```python
from build123d import *

# Parameters (mm, degrees)
F0_W      = 14
F0_H      = 58
F1_DEPTH  = 5
F3_DEPTH  = 25
F5_W      = 23
F5_H      = 3.5
F6_DEPTH  = 19.5
F7_W      = 14
F7_H      = 5
F8_DEPTH  = 8
F10_DEPTH = 12


with BuildPart() as f1:
    # F0 (on Top) → F1 (new body)
    with BuildSketch(Plane.XY):
        with Locations((7, 29)):
            Rectangle(F0_W, F0_H)
    extrude(amount=F1_DEPTH)

    # F2 (on face) → F3 (cut)
    with BuildSketch(Plane.XY.offset(5)):
        with BuildLine():
            ThreePointArc((8.5, 26.9), (8.0606601718, 27.9606601718), (7, 28.4))
            Line((7, 28.4), (7, 26.9))
            Line((7, 26.9), (8.5, 26.9))
        make_face()
        with BuildLine():
            Line((7, 26.9), (7, 28.4))
            ThreePointArc((7, 28.4), (5.9393398282, 27.9606601718), (5.5, 26.9))
            Line((5.5, 26.9), (7, 26.9))
        make_face()
        with BuildLine():
            Line((7, 25.4), (7, 26.9))
            Line((7, 26.9), (5.5, 26.9))
            ThreePointArc((5.5, 26.9), (5.9393398282, 25.8393398282), (7, 25.4))
        make_face()
        with BuildLine():
            Line((8.5, 26.9), (7, 26.9))
            Line((7, 26.9), (7, 25.4))
            ThreePointArc((7, 25.4), (8.0606601718, 25.8393398282), (8.5, 26.9))
        make_face()
        with BuildLine():
            ThreePointArc((8.5, 6.6), (8.0606601718, 7.6606601718), (7, 8.1))
            Line((7, 8.1), (7, 6.6))
            Line((7, 6.6), (8.5, 6.6))
        make_face()
        with BuildLine():
            Line((7, 6.6), (7, 8.1))
            ThreePointArc((7, 8.1), (5.9393398282, 5.5393398282), (8.5, 6.6))
            Line((8.5, 6.6), (7, 6.6))
        make_face()
    extrude(amount=-F3_DEPTH, mode=Mode.SUBTRACT)

    # F5 (on offset) → F6 (join)
    with BuildSketch(Plane(origin=(0, 55.5, 0), x_dir=(-1, 0, 0), z_dir=(0, 1, 0))):
        with Locations((-7, 10.25)):
            Rectangle(F5_W, F5_H)
        Polygon((-18.5, 0), (0, 0), (4.5, 0), (4.5, 8.5), (-18.5, 8.5), align=None)
    extrude(amount=-F6_DEPTH)

    # F7 (on face) → F8 (cut)
    with BuildSketch(Plane(origin=(0, 58, 0), x_dir=(-1, 0, 0), z_dir=(0, 1, 0))):
        with Locations((-7, 2.5)):
            Rectangle(F7_W, F7_H)
        Polygon((-18.5, 0), (-14, 0), (-14, 5), (0, 5), (0, 8.5), (-18.5, 8.5), align=None)
        Polygon((0, 5), (0, 0), (4.5, 0), (4.5, 8.5), (0, 8.5), align=None)
        Polygon((-18.5, 8.5), (0, 8.5), (4.5, 8.5), (4.5, 12), (-18.5, 12), align=None)
    extrude(amount=-F8_DEPTH, mode=Mode.SUBTRACT)

    # F9 (on face) → F10 (cut)
    with BuildSketch(Plane(origin=(0, 50, 0), x_dir=(-1, 0, 0), z_dir=(0, 1, 0))):
        with BuildLine():
            ThreePointArc((-10, 6), (-10.3661165235, 6.8838834765), (-11.25, 7.25))
            Line((-11.25, 7.25), (-11.25, 6))
            Line((-11.25, 6), (-12.5, 6))
            ThreePointArc((-12.5, 6), (-11.25, 4.75), (-10, 6))
        make_face()
        with BuildLine():
            Line((-11.25, 6), (-11.25, 7.25))
            ThreePointArc((-11.25, 7.25), (-12.1338834765, 6.8838834765), (-12.5, 6))
            Line((-12.5, 6), (-11.25, 6))
        make_face()
        with BuildLine():
            ThreePointArc((-1.5, 6), (-1.8661165235, 6.8838834765), (-2.75, 7.25))
            Line((-2.75, 7.25), (-2.75, 6))
            Line((-2.75, 6), (-1.5, 6))
        make_face()
        with BuildLine():
            Line((-2.75, 6), (-2.75, 7.25))
            ThreePointArc((-2.75, 7.25), (-3.6338834765, 5.1161165235), (-1.5, 6))
            Line((-1.5, 6), (-2.75, 6))
        make_face()
    extrude(amount=-F10_DEPTH, mode=Mode.SUBTRACT)


solid = f1.part
```
Geometry: final body of the model. Coordinates: model frame, mm. A direction names the side the tool comes from. Round coordinates to 2 decimals unless told otherwise and drop trailing zeros. Order: outer loops, then holes, each group sorted by start corner. A loop starts at its lowest first (then second) coordinate and runs counter-clockwise, first axis right, second up. Notation, with made-up numbers: (89, 70) -> (140, 70) arc R16 cw to (140, 95) -> close; hole circle Ø7 at (0.5, 21). An arc over 180 degrees is marked (long way). Use one line per item in the form item = value.
(1) Ray query, probe 1 along X at (y, z) = (46.5, 6); probe 2 along Y at (x, z) = (7, 2.25); probe 3 along Z at (x, y) = (2.75, 41.5). Return the intervals inside material, ascending. Write a range as [from, to].
Results list:
probe_1 = [-4.5, 1.5], [4, 10], [12.5, 18.5]
probe_2 = [0, 5.1], [8.1, 25.4], [28.4, 50]
probe_3 = [0, 4.75], [7.25, 12]
(2) First-contact query: pin 1 Ø1.2 at (x, z) = (11.5, 5.5) entering from +Y; pin 2 Ø6 at (x, y) = (14.5, 31.5) entering from +Z; pin 3 Ø1.5 at (y, z) = (21, 5.5) entering from +X; pin 4 Ø5 at (y, z) = (21, 9) entering from -X. Flat tips, straight axial feed; report the tip coordinate or a pass-through.
Results list:
pin_1 = 38
pin_2 = 5
pin_3 = 14
pin_4 = through
(3) Draft query along Z for faces 1 (the face through (7, 43, 12)), 2 (the face through (3, 38, 6)), 3 (the face through (7, 50, 6)). Return one class per face: pulls with the +Z half, pulls with the -Z half, needs draft (parallel to the pull), parting line crosses it, or undercut.
Results list:
face_1 = pulls with the +Z half
face_2 = undercut
face_3 = needs draft
(4) Access query for faces 4 (the face through (11, 38, 6)), 5 (the face through (7, 18, 5)), 6 (the face through (14, 18, 2)), 7 (the face through (0, 18, 2)). Directions: +Z, -Z, +X, -X, +Y, -Y. A direction counts if a zero-diameter tool reaches every point of the face in a straight line with its end or side. Return the directions, or none.
Results list:
face_4 = +Y
face_5 = +Z, +X, -X, -Y
face_6 = +Z, -Z, +X, -Y
face_7 = +Z, -Z, -X, -Y
(5) Section D-D on y = 20.5. Return loops of the section in (x, z), and give its area (3 significant figures).
Results list:
outline = (0, 0) -> (14, 0) -> (14, 5) -> (0, 5) -> close
area = 70.0 mm^2
(6) Section A-A on y = 42. Return loops of the section in (x, z).
Results list:
outline = (-4.5, 0) -> (18.5, 0) -> (18.5, 12) -> (-4.5, 12) -> close; hole circle Ø2.5 at (2.75, 6); hole circle Ø2.5 at (11.25, 6)
(7) Section C-C on x = -1. Return loops of the section in (y, z).
Results list:
outline = (36, 0) -> (50, 0) -> (50, 12) -> (36, 12) -> close
(8) Section B-B on z = 3.75. Return loops of the section in (x, y).
Results list:
outline = (-4.5, 36) -> (0, 36) -> (0, 0) -> (14, 0) -> (14, 36) -> (18.5, 36) -> (18.5, 50) -> (-4.5, 50) -> close; hole circle Ø3 at (7, 6.6); hole circle Ø3 at (7, 26.9)
